Model file for the job. Use its own axes, mm. A direction names the side the tool comes from. Round coordinates to 2 decimals unless told otherwise and drop trailing zeros. Put each result on its own line as item: value. Start each with the question number.
Q1. Flat gauge pins, fed straight in: P1, Ø0.5, axis at x = 114, z = 9, coming from the -Y side; P2, Ø1.4, axis at x = 85.5, z = -0.5, coming from the -Y side; P3, Ø4, axis at x = 100.5, y = 0, coming from the -Z side. Where does each tip first touch, or does it go through?
Q2. Pull direction Y, two halves, no side cores. Call faces 1 (the face through (84, -6, 10)), 2 (the face through (84, -10, -6)), 3 (the face through (83.81, 5.33, 4.27)), 4 (the face through (83.81, 4.32, 5.38)): released by +Y, released by -Y, zero draft, split by the parting line, or undercut.
Q3. 3-axis set-ups, long thin cutter, end or side, ignore diameter. For faces 5 (the face through (84, 0, -3.659)), 6 (the face through (84, -3.659, 0)), 7 (the face through (83.81, -5.33, -4.27)), 8 (the face through (84, 10, -6)), 9 (the face through (84, -6, -10)): which of +Z, -Z, +X, -X, +Y, -Y reach the whole face in a straight line?
Q4. Probe L1, parallel to Y at x = 106.5, z = -0.25; L2, parallel to Z at x = 106, y = 0; L3, parallel to Y at x = 12, z = -7.5. List the from-to ranges inside material, lowest first.
from build123d import *

# Parameters (mm, degrees)
F_20_SERIES_20_2020_1_DEPTH = 170


with BuildPart() as part:
    # Sketch11 → 20_series 20-2020(1) (new body)
    with BuildSketch(Plane(origin=(0, 0, 0), x_dir=(0, 0, -1), z_dir=(1, 0, 0))):
        with BuildLine():
            Line((9.0094, 2.6289), (9.492, 2.6289))
            ThreePointArc((9.492, 2.6289), (9.851210245, 2.777689755), (10, 3.1369))
            Line((10, 3.1369), (10, 8.5014))
            ThreePointArc((10, 8.5014), (9.561070222, 9.561070222), (8.5014, 10))
            Line((8.5014, 10), (3.1369, 10))
            ThreePointArc((3.1369, 10), (2.777689755, 9.851210245), (2.6289, 9.492))
            Line((2.6289, 9.492), (2.6289, 9.0094))
            ThreePointArc((2.6289, 9.0094), (2.777689755, 8.650189755), (3.1369, 8.5014))
            Line((3.1369, 8.5014), (5.4864, 8.5014))
            ThreePointArc((5.4864, 8.5014), (5.845610245, 8.352610245), (5.9944, 7.9934))
            Line((5.9944, 7.9934), (5.9944, 7.264490712))
            ThreePointArc((5.9944, 7.264490712), (5.955730803, 7.070087528), (5.845610245, 6.905280467))
            Line((5.845610245, 6.905280467), (2.747686782, 3.807357004))
            ThreePointArc((2.747686782, 3.807357004), (2.582879721, 3.697236446), (2.388476537, 3.658567249))
            Line((2.388476537, 3.658567249), (-2.388476537, 3.658567249))
            ThreePointArc((-2.388476537, 3.658567249), (-2.582879721, 3.697236446), (-2.747686782, 3.807357004))
            Line((-2.747686782, 3.807357004), (-5.845610245, 6.905280467))
            ThreePointArc((-5.845610245, 6.905280467), (-5.955730803, 7.070087528), (-5.9944, 7.264490712))
            Line((-5.9944, 7.264490712), (-5.9944, 7.9934))
            ThreePointArc((-5.9944, 7.9934), (-5.845610245, 8.352610245), (-5.4864, 8.5014))
            Line((-5.4864, 8.5014), (-3.1369, 8.5014))
            ThreePointArc((-3.1369, 8.5014), (-2.777689755, 8.650189755), (-2.6289, 9.0094))
            Line((-2.6289, 9.0094), (-2.6289, 9.492))
            ThreePointArc((-2.6289, 9.492), (-2.777689755, 9.851210245), (-3.1369, 10))
            Line((-3.1369, 10), (-8.5014, 10))
            ThreePointArc((-8.5014, 10), (-9.561070222, 9.561070222), (-10, 8.5014))
            Line((-10, 8.5014), (-10, 3.1369))
            ThreePointArc((-10, 3.1369), (-9.851210245, 2.777689755), (-9.492, 2.6289))
            Line((-9.492, 2.6289), (-9.0094, 2.6289))
            ThreePointArc((-9.0094, 2.6289), (-8.650189755, 2.777689755), (-8.5014, 3.1369))
            Line((-8.5014, 3.1369), (-8.5014, 5.4864))
            ThreePointArc((-8.5014, 5.4864), (-8.352610245, 5.845610245), (-7.9934, 5.9944))
            Line((-7.9934, 5.9944), (-7.264490712, 5.9944))
            ThreePointArc((-7.264490712, 5.9944), (-7.070087528, 5.955730803), (-6.905280467, 5.845610245))
            Line((-6.905280467, 5.845610245), (-3.807357004, 2.747686782))
            ThreePointArc((-3.807357004, 2.747686782), (-3.697236446, 2.582879721), (-3.658567249, 2.388476537))
            Line((-3.658567249, 2.388476537), (-3.658567249, -2.388476537))
            ThreePointArc((-3.658567249, -2.388476537), (-3.697236446, -2.582879721), (-3.807357004, -2.747686782))
            Line((-3.807357004, -2.747686782), (-6.905280467, -5.845610245))
            ThreePointArc((-6.905280467, -5.845610245), (-7.070087528, -5.955730803), (-7.264490712, -5.9944))
            Line((-7.264490712, -5.9944), (-7.9934, -5.9944))
            ThreePointArc((-7.9934, -5.9944), (-8.352610245, -5.845610245), (-8.5014, -5.4864))
            Line((-8.5014, -5.4864), (-8.5014, -3.1369))
            ThreePointArc((-8.5014, -3.1369), (-8.650189755, -2.777689755), (-9.0094, -2.6289))
            Line((-9.0094, -2.6289), (-9.492, -2.6289))
            ThreePointArc((-9.492, -2.6289), (-9.851210245, -2.777689755), (-10, -3.1369))
            Line((-10, -3.1369), (-10, -8.5014))
            ThreePointArc((-10, -8.5014), (-9.561070222, -9.561070222), (-8.5014, -10))
            Line((-8.5014, -10), (-3.1369, -10))
            ThreePointArc((-3.1369, -10), (-2.777689755, -9.851210245), (-2.6289, -9.492))
            Line((-2.6289, -9.492), (-2.6289, -9.0094))
            ThreePointArc((-2.6289, -9.0094), (-2.777689755, -8.650189755), (-3.1369, -8.5014))
            Line((-3.1369, -8.5014), (-5.4864, -8.5014))
            ThreePointArc((-5.4864, -8.5014), (-5.845610245, -8.352610245), (-5.9944, -7.9934))
            Line((-5.9944, -7.9934), (-5.9944, -7.264490712))
            ThreePointArc((-5.9944, -7.264490712), (-5.955730803, -7.070087528), (-5.845610245, -6.905280467))
            Line((-5.845610245, -6.905280467), (-2.747686782, -3.807357004))
            ThreePointArc((-2.747686782, -3.807357004), (-2.582879721, -3.697236446), (-2.388476537, -3.658567249))
            Line((-2.388476537, -3.658567249), (2.388476537, -3.658567249))
            ThreePointArc((2.388476537, -3.658567249), (2.582879721, -3.697236446), (2.747686782, -3.807357004))
            Line((2.747686782, -3.807357004), (5.845610245, -6.905280467))
            ThreePointArc((5.845610245, -6.905280467), (5.955730803, -7.070087528), (5.9944, -7.264490712))
            Line((5.9944, -7.264490712), (5.9944, -7.9934))
            ThreePointArc((5.9944, -7.9934), (5.845610245, -8.352610245), (5.4864, -8.5014))
            Line((5.4864, -8.5014), (3.1369, -8.5014))
            ThreePointArc((3.1369, -8.5014), (2.777689755, -8.650189755), (2.6289, -9.0094))
            Line((2.6289, -9.0094), (2.6289, -9.492))
            ThreePointArc((2.6289, -9.492), (2.777689755, -9.851210245), (3.1369, -10))
            Line((3.1369, -10), (8.5014, -10))
            ThreePointArc((8.5014, -10), (9.561070222, -9.561070222), (10, -8.5014))
            Line((10, -8.5014), (10, -3.1369))
            ThreePointArc((10, -3.1369), (9.851210245, -2.777689755), (9.492, -2.6289))
            Line((9.492, -2.6289), (9.0094, -2.6289))
            ThreePointArc((9.0094, -2.6289), (8.650189755, -2.777689755), (8.5014, -3.1369))
            Line((8.5014, -3.1369), (8.5014, -5.4864))
            ThreePointArc((8.5014, -5.4864), (8.352610245, -5.845610245), (7.9934, -5.9944))
            Line((7.9934, -5.9944), (7.264490712, -5.9944))
            ThreePointArc((7.264490712, -5.9944), (7.070087528, -5.955730803), (6.905280467, -5.845610245))
            Line((6.905280467, -5.845610245), (3.807357004, -2.747686782))
            ThreePointArc((3.807357004, -2.747686782), (3.697236446, -2.582879721), (3.658567249, -2.388476537))
            Line((3.658567249, -2.388476537), (3.658567249, 2.388476537))
            ThreePointArc((3.658567249, 2.388476537), (3.697236446, 2.582879721), (3.807357004, 2.747686782))
            Line((3.807357004, 2.747686782), (6.905280467, 5.845610245))
            ThreePointArc((6.905280467, 5.845610245), (7.070087528, 5.955730803), (7.264490712, 5.9944))
            Line((7.264490712, 5.9944), (7.9934, 5.9944))
            ThreePointArc((7.9934, 5.9944), (8.352610245, 5.845610245), (8.5014, 5.4864))
            Line((8.5014, 5.4864), (8.5014, 3.1369))
            ThreePointArc((8.5014, 3.1369), (8.650189755, 2.777689755), (9.0094, 2.6289))
        make_face()
        with BuildLine():
            Line((-2.296558466, 2.121727546), (-2.121727546, 2.296558466))
            ThreePointArc((-2.121727546, 2.296558466), (-1.459775814, 2.520126613), (-0.880635441, 2.129282347))
            ThreePointArc((-0.880635441, 2.129282347), (-0.755121693, 2.019456424), (-0.588548999, 2.011151493))
            ThreePointArc((-0.588548999, 2.011151493), (0, 2.0955), (0.588548999, 2.011151493))
            ThreePointArc((0.588548999, 2.011151493), (0.755121693, 2.019456424), (0.880635441, 2.129282347))
            ThreePointArc((0.880635441, 2.129282347), (1.459775814, 2.520126613), (2.121727546, 2.296558466))
            Line((2.121727546, 2.296558466), (2.296558466, 2.121727546))
            ThreePointArc((2.296558466, 2.121727546), (2.520126613, 1.459775814), (2.129282347, 0.880635441))
            ThreePointArc((2.129282347, 0.880635441), (2.019456424, 0.755121693), (2.011151493, 0.588548999))
            ThreePointArc((2.011151493, 0.588548999), (2.0955, 0), (2.011151493, -0.588548999))
            ThreePointArc((2.011151493, -0.588548999), (2.019456424, -0.755121693), (2.129282347, -0.880635441))
            ThreePointArc((2.129282347, -0.880635441), (2.520126613, -1.459775814), (2.296558466, -2.121727546))
            Line((2.296558466, -2.121727546), (2.121727546, -2.296558466))
            ThreePointArc((2.121727546, -2.296558466), (1.459775814, -2.520126613), (0.880635441, -2.129282347))
            ThreePointArc((0.880635441, -2.129282347), (0.755121693, -2.019456424), (0.588548999, -2.011151493))
            ThreePointArc((0.588548999, -2.011151493), (0, -2.0955), (-0.588548999, -2.011151493))
            ThreePointArc((-0.588548999, -2.011151493), (-0.755121693, -2.019456424), (-0.880635441, -2.129282347))
            ThreePointArc((-0.880635441, -2.129282347), (-1.459775814, -2.520126613), (-2.121727546, -2.296558466))
            Line((-2.121727546, -2.296558466), (-2.296558466, -2.121727546))
            ThreePointArc((-2.296558466, -2.121727546), (-2.520126613, -1.459775814), (-2.129282347, -0.880635441))
            ThreePointArc((-2.129282347, -0.880635441), (-2.019456424, -0.755121693), (-2.011151493, -0.588548999))
            ThreePointArc((-2.011151493, -0.588548999), (-2.0955, 0), (-2.011151493, 0.588548999))
            ThreePointArc((-2.011151493, 0.588548999), (-2.019456424, 0.755121693), (-2.129282347, 0.880635441))
            ThreePointArc((-2.129282347, 0.880635441), (-2.520126613, 1.459775814), (-2.296558466, 2.121727546))
        make_face(mode=Mode.SUBTRACT)
    extrude(amount=F_20_SERIES_20_2020_1_DEPTH)


solid = part.part
Ans:
1. P1: stops at y = -9.98
1. P2: stops at y = -3.66
1. P3: stops at z = -3.66
2. face 1: zero draft
2. face 2: released by -Y
2. face 3: undercut
2. face 4: undercut
3. face 5: -Z, +X, -X
3. face 6: +X, -X, -Y
3. face 7: +X, -X
3. face 8: +Z, -Z, +X, -X, +Y
3. face 9: -Z, +X, -X, +Y, -Y
4. L1: y = -3.66 to -2.08, 2.08 to 3.66
4. L2: z = -3.66 to -2.1, 2.1 to 3.66
4. L3: y = -10 to -5.99, 5.99 to 10
